```python
from build123d import *

# Parameters (mm, degrees)
EXTRUDE_1_DEPTH          = 40
SKETCH_2_W               = 25
SKETCH_2_H               = 25
EXTRUDE_2_DEPTH          = 5
SKETCH_3_W               = 20
SKETCH_3_H               = 5
CUT_EXTRUDE_1_DEPTH      = 20
CUT_EXTRUDE_2_DEPTH      = 50.497474683
CUT_EXTRUDE_2_DEPTH_BACK = 50.497474683
SKETCH_4_W               = 7.5
SKETCH_4_H               = 45


with BuildPart() as part:
    # 스케치1 → 보스-돌출1 (new body)
    with BuildSketch(Plane(origin=(0, 0, 0), x_dir=(1, 0, 0), z_dir=(0, 1, 0))):
        Polygon((0, 0), (25, 0), (25, 10), (10, 10), (10, 25), (0, 25), align=None)
    extrude(amount=EXTRUDE_1_DEPTH)

    # 스케치2 → 보스-돌출2 (add)
    with BuildSketch(Plane.XZ):
        with Locations((12.5, -12.5)):
            Rectangle(SKETCH_2_W, SKETCH_2_H)
    extrude(amount=EXTRUDE_2_DEPTH)

    # 스케치3 → 컷-돌출1 (cut)
    with BuildSketch(Plane(origin=(0, 0, -25), x_dir=(-1, 0, 0), z_dir=(0, 0, -1))):
        with Locations((-15, 32.5)):
            Rectangle(SKETCH_3_W, SKETCH_3_H)
    extrude(amount=-CUT_EXTRUDE_1_DEPTH, mode=Mode.SUBTRACT)

    # 스케치4 → 컷-돌출2 (cut, two sides: drawn at the far end of the back side and taken through both)
    with BuildSketch(Plane(origin=(10, 0, 0), x_dir=(0, 0, -1), z_dir=(1, 0, 0)).offset(-CUT_EXTRUDE_2_DEPTH_BACK)):
        with Locations((21.25, 17.5)):
            Rectangle(SKETCH_4_W, SKETCH_4_H)
    extrude(amount=CUT_EXTRUDE_2_DEPTH + CUT_EXTRUDE_2_DEPTH_BACK, mode=Mode.SUBTRACT)


solid = part.part
```
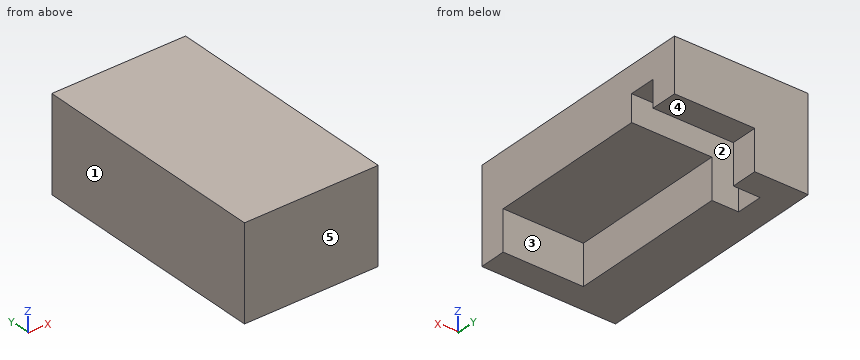
The model under review builds one solid part; all positions refer to its coordinate system, in mm. Face numbers are marked on the shaded views. A direction names the side the tool comes from. Round coordinates to 2 decimals unless told otherwise and drop trailing zeros. Loops run counter-clockwise (first coordinate to the right, second up) from the corner with the lowest first, then second, coordinate; pieces in that order, holes last. Notation, with made-up numbers: (75, 5) - (96, 5) arc R11 ccw to (96, 13) - close; hole circle Ø1 at (87.25, -5). An arc over 180 degrees is marked (long way). Write each question's results on one line, items separated by ' | '. Start each with the question number.
Q1. Take a section at A-A on x = 10.75. Give the boundary of the cut face in (y, z).
Q2. Draft analysis for pull direction Y (two halves, no side actions). For the marked faces 1, 2 and 3, state which applies: pulls with the +Y half, pulls with the -Y half, needs draft (parallel to the pull), parting line crosses it, or undercut.
Q3. Take a section at C-C on y = 26.5. Give the boundary of the cut face in (x, z), plus the area to 3 significant figures.
Q4. Take a section at D-D on z = -9.5. Give the boundary of the cut face in (x, y).
Q5. Insertion check: P1, Ø5.5, axis at x = 13, y = 33, coming from the -Z side; P2, Ø8, axis at x = 19, z = -15.5, coming from the +Y side; P3, Ø5.5, axis at y = 37, z = -13.5, coming from the +X side. Each pin has a flat end and moves straight along its axis. Give the tip position at first contact, or say it passes through.
Q6. Take a section at B-B on z = -12.5. Give the boundary of the cut face in (x, y), plus the area to 3 significant figures.
Q7. Wall thickness on line 1 along Y through (x, z) = (23.75, -8.5); line 2 along X through (y, z) = (37, -11.75); line 3 along X through (y, z) = (30.5, -12.25): over which ranges is each line inside the solid? List them lowest first. Write a range as [from, to].
Q8. Tool access review of the marked faces 4 and 5: name each direction out of +Z, -Z, +X, -X, +Y, -Y from which nothing blocks a thin tool from reaching the whole face with its end or side.
Data:
1) outline: (-5, -17.5) - (0, -17.5) - (0, -10) - (30, -10) - (30, -5) - (35, -5) - (35, -10) - (40, -10) - (40, 0) - (-5, 0) - close
2) face 1: needs draft | face 2: undercut | face 3: pulls with the +Y half
3) outline: (0, -17.5) - (10, -17.5) - (10, -10) - (25, -10) - (25, 0) - (0, 0) - close | area: 325 mm²
4) outline: (0, -5) - (25, -5) - (25, 30) - (5, 30) - (5, 35) - (25, 35) - (25, 40) - (0, 40) - close
5) P1: stops at z = -10 | P2: stops at y = 0 | P3: stops at x = 10
6) outline: (0, -5) - (25, -5) - (25, 0) - (10, 0) - (10, 30) - (5, 30) - (5, 35) - (10, 35) - (10, 40) - (0, 40) - close | area: 500 mm²
7) line 1: y = [-5, 30], [35, 40] | line 2: x = [0, 10] | line 3: x = [0, 5]
8) face 4: -Z, +X, +Y | face 5: +Z, -Z, +X, -X, -Y
